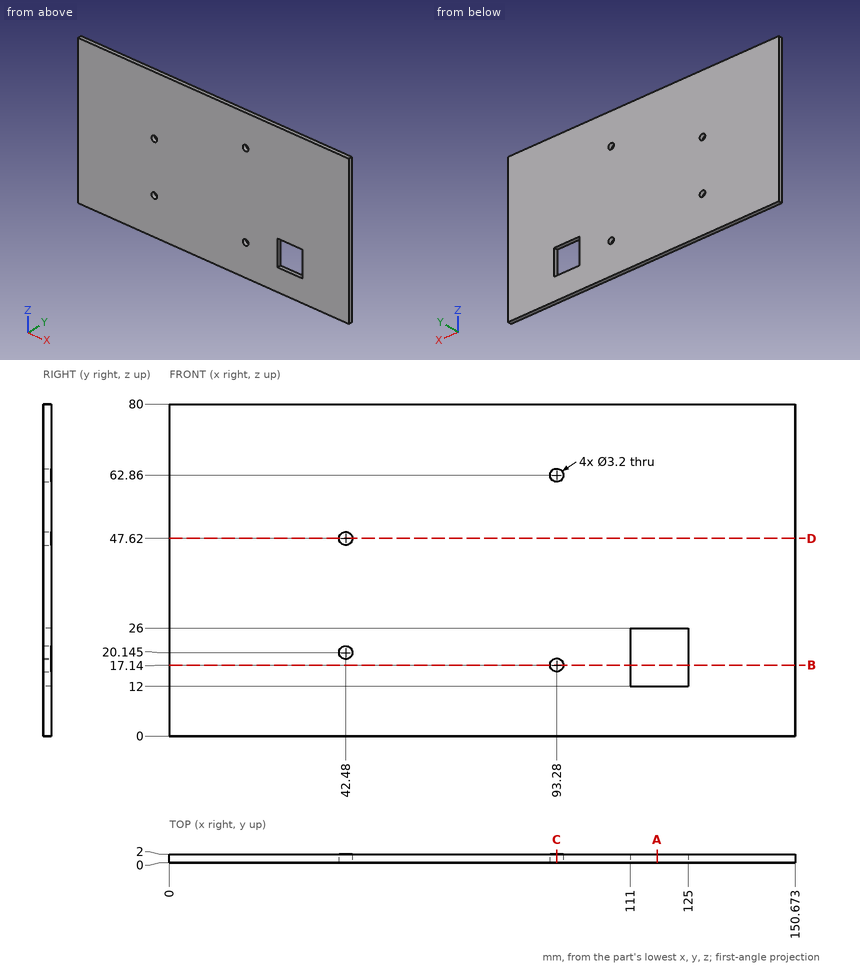
The figure shows three views and two pictorial views of one solid part (mm, origin at its lowest corner). Answer the questions. Give positions to 0.01 mm unless a question says otherwise; leave off trailing zeros. Order: outer loops, then holes, each group sorted by start corner. A loop starts at its lowest first (then second) coordinate and runs counter-clockwise, first axis right, second up. Notation, with made-up numbers: (52.5, 24.5) - (110.5, 24.5) arc R17 cw to (110.5, 51.5) - close; hole circle Ø7 at (27, -5.75). An arc over 180 degrees is marked (long way). Answer as CSV lines item,"result".
Q1. A cutting plane is placed at A-A, the plane x = 117.5. Determine the outline of the cut face in (y, z), and give its area (3 significant figures).
Answer key:
outline,"(0, 0) - (2, 0) - (2, 12) - (0, 12) - close; (0, 26) - (2, 26) - (2, 80) - (0, 80) - close"
area,"132 mm^2"
Q2. Straight lines are drawn through the part: L1, parallel to Z at x = 42.48, y = 0.4 (1 decimal); L2, parallel to Z at x = 93.28, y = 0.85; L3, parallel to X at y = 1, z = 23.5. For each, find the intervals that lie inside material, in ascending order.
Answer key:
L1,"z = 0 to 18.5, 21.7 to 46, 49.2 to 80"
L2,"z = 0 to 15.54, 18.74 to 61.26, 64.46 to 80"
L3,"x = 0 to 111, 125 to 150.67"
Q3. A cutting plane is placed at B-B, the plane z = 17.14. Determine the outline of the cut face in (x, y), and give its area (3 significant figures).
Answer key:
outline,"(0, 0) - (91.68, 0) - (91.68, 2) - (0, 2) - close; (94.88, 0) - (111, 0) - (111, 2) - (94.88, 2) - close; (125, 0) - (150.67, 0) - (150.67, 2) - (125, 2) - close"
area,"267 mm^2"
Q4. A cutting plane is placed at D-D, the plane z = 47.62. Determine the outline of the cut face in (x, y).
Answer key:
outline,"(0, 0) - (40.88, 0) - (40.88, 2) - (0, 2) - close; (44.08, 0) - (150.67, 0) - (150.67, 2) - (44.08, 2) - close"
Q5. A cutting plane is placed at C-C, the plane x = 93.28. Determine the outline of the cut face in (y, z), and give its area (3 significant figures).
Answer key:
outline,"(0, 0) - (2, 0) - (2, 15.54) - (0, 15.54) - close; (0, 18.74) - (2, 18.74) - (2, 61.26) - (0, 61.26) - close; (0, 64.46) - (2, 64.46) - (2, 80) - (0, 80) - close"
area,"147 mm^2"
